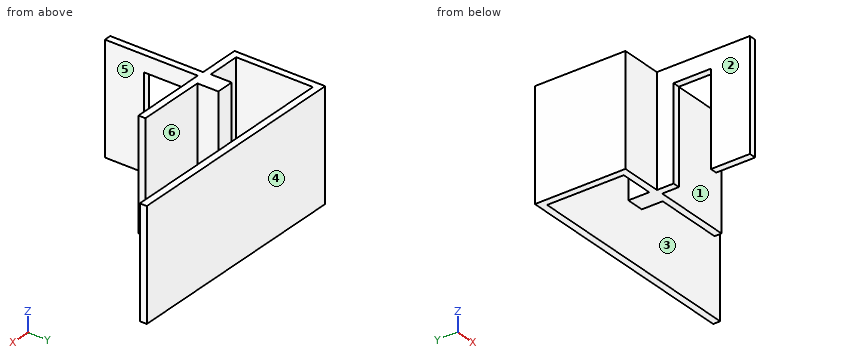
from build123d import *

# Parameters (mm, degrees)
F1_DEPTH = 235
F2_W     = 80
F2_H     = 200
F3_DEPTH = 104.001


with BuildPart() as f1:
    # F0 (on Top) → F1 (new body)
    with BuildSketch(Plane.XY):
        Polygon((-117.413361, 188.052049), (372.586639, 188.052049), (372.586639, 203.052049), (-132.413361, 203.052049), (-132.413361, 8.052049), (-43.413361, 8.052049), (-43.413361, -191.947951), (-28.413361, -191.947951), (-28.413361, 8.052049), (139.586639, 8.052049), (139.586639, 23.052049), (-7.413361, 23.052049), (-7.413361, 68.052049), (-45.413361, 68.052049), (-45.413361, 23.052049), (-117.413361, 23.052049), align=None)
    extrude(amount=F1_DEPTH)

    # F2 (on face) → F3 (cut, through all)
    with BuildSketch(Plane.YZ.offset(-28.413361)):
        with Locations((-67.947951, 100)):
            Rectangle(F2_W, F2_H)
    extrude(amount=-F3_DEPTH, mode=Mode.SUBTRACT)


solid = f1.part
Read the model definition and answer for the solid it produces. Units are mm, in the model's axes. Face numbers are marked on the shaded views. A direction names the side the tool comes from. Round coordinates to 2 decimals unless told otherwise and drop trailing zeros. Write each loop counter-clockwise with the first axis right and the second up, starting at its lowest first coordinate (ties: lowest second). Pieces come first, ordered by that corner, then holes. Notation, with made-up numbers: (-27, 80) - (21, 80) arc R33 cw to (21, 117) - close; hole circle Ø4 at (33, -10). An arc over 180 degrees is marked (long way). Use a Markdown table: item, result.
(1) The part is cut by section C-C (z = 55). Write down the section's boundary in (x, y).
Reported:
| item | result |
|---|---|
| outline | (-132.41, 8.05) - (-43.41, 8.05) - (-43.41, -27.95) - (-28.41, -27.95) - (-28.41, 8.05) - (139.59, 8.05) - (139.59, 23.05) - (-7.41, 23.05) - (-7.41, 68.05) - (-45.41, 68.05) - (-45.41, 23.05) - (-117.41, 23.05) - (-117.41, 188.05) - (372.59, 188.05) - (372.59, 203.05) - (-132.41, 203.05) - close; (-43.41, -191.95) - (-28.41, -191.95) - (-28.41, -107.95) - (-43.41, -107.95) - close |
(2) The mould has two halves that part along Y. Classify the marked faces 4, 5 and 6: released by +Y, released by -Y, zero draft, split by the parting line, or undercut.
Reported:
| item | result |
|---|---|
| face 4 | released by +Y |
| face 5 | zero draft |
| face 6 | undercut |
(3) Straight lines are drawn through the part: line 1 along Y through (x, z) = (45.5, 165.5); line 2 along X through (y, z) = (-12.5, 171); line 3 along X through (y, z) = (83, 111.5). For each, find the intervals that lie inside material, in ascending order. Write a range as [from, to].
Reported:
| item | result |
|---|---|
| line 1 | [8.05, 23.05], [188.05, 203.05] |
| line 2 | [-43.41, -28.41] |
| line 3 | [-132.41, -117.41] |
(4) The part is cut by section A-A (y = 44). Write down the section's boundary in (x, z).
Reported:
| item | result |
|---|---|
| outline | (-132.41, 0) - (-117.41, 0) - (-117.41, 235) - (-132.41, 235) - close; (-45.41, 0) - (-7.41, 0) - (-7.41, 235) - (-45.41, 235) - close |
(5) Each of these flat-tipped pins is pushed along its axis until it touches: pin 1 Ø1.5 at (x, z) = (288, 98.5) entering from -Y; pin 2 Ø3 at (x, z) = (-15, 148) entering from -Y; pin 3 Ø12 at (x, y) = (-38, -61.5) entering from -Z. Where does it stop, or does it pass through?
Reported:
| item | result |
|---|---|
| pin 1 | y = 188.05 |
| pin 2 | y = 8.05 |
| pin 3 | z = 200 |
(6) Which of the six approach directions +Z, -Z, +X, -X, +Y, -Y give full straight-line access (tool end or side, diameter ignored) to the marked faces 1, 2 and 3?
Reported:
| item | result |
|---|---|
| face 1 | +Z, -Z, +X, -Y |
| face 2 | +Z, -Z, -X, -Y |
| face 3 | +Z, -Z, +X |
(7) The part is cut by section B-B (x = -85). Write down the section's boundary in (y, z).
Reported:
| item | result |
|---|---|
| outline | (8.05, 0) - (23.05, 0) - (23.05, 235) - (8.05, 235) - close; (188.05, 0) - (203.05, 0) - (203.05, 235) - (188.05, 235) - close |
(8) The part is cut by section D-D (y = -99). Write down the section's boundary in (x, z), then the cut area to 3 significant figures.
Reported:
| item | result |
|---|---|
| outline | (-43.41, 200) - (-28.41, 200) - (-28.41, 235) - (-43.41, 235) - close |
| area | 525 mm2 |
